Could you check a few things on this model? Use its own coordinates, in mm. A direction names the side the tool comes from. Coordinates: 2 decimals unless noted, no trailing zeros. Order: outer loops, then holes, each group sorted by start corner. A loop starts at its lowest first (then second) coordinate and runs counter-clockwise, first axis right, second up. Notation, with made-up numbers: M 62,39 L 87,39 A26 cw 87,74 Z; hole C 85.25,-4 d4. An arc over 180 degrees is marked long. One line per question, with ' | ' between items. Start each with the question number.
from build123d import *

# Parameters (mm, degrees)
CYLINDER157_R     = 2
CYLINDER157_DEPTH = 10
EXTRUDE038_DEPTH  = 28


with BuildPart() as cylinder157:
    # Cylinder157 → Cylinder157 (new body)
    with BuildSketch(Plane(origin=(0, -238, -147.25), x_dir=(1, 0, 0), z_dir=(0, -1, 0))):
        Circle(CYLINDER157_R)
    extrude(amount=CYLINDER157_DEPTH)


with BuildPart() as logoattach001:
    # Sketch056 → Extrude038 (new body)
    with BuildSketch(Plane.XY):
        with BuildLine():
            ThreePointArc((-20, -241.335918), (0, -243.5), (20, -241.335918))
            Line((20, -237.335918), (20, -241.335918))
            Line((-20, -237.335918), (20, -237.335918))
            Line((-20, -241.335918), (-20, -237.335918))
        make_face()
    extrude(amount=EXTRUDE038_DEPTH)


with BuildPart() as logoattach001_1:
    # Extrude038 placement: moved
    add(logoattach001.part.moved(Location((0, 0, -160))))

    # Fusion105: union Cylinder157
    add(cylinder157.part)


solid = logoattach001_1.part
(1) On a 3-axis mill with a long thin cutter (end or side, diameter ignored), from which of +Z, -Z, +X, -X, +Y, -Y can I reach the whole of each face in a straight line? I mean faces 1 (the flat face through (0, -240, -160)), 2 (the cylindrical face through (0.923, -245.707, -149.024)). Say none if no direction works.
(2) Imagine slicing it at B-B, the plane z = -147.25. Write out the boundary of the cut face in (x, y), plus the area to 3 significant figures.
(3) Imagine slicing it at A-A, the plane x = 0. Write out the boundary of the cut face in (y, z).
(4) For P1, Ø10, axis at x = -11, z = -139.5, coming from the -Y side; P2, Ø3, axis at y = -242.5, z = -146, coming from the +X side, each with a flat end and sliding along its axis, tell me the tip position at first contact or that it passes through.
(5) If I drill on line 1 along Y through (x, z) = (7.5, -138); line 2 along Y through (x, z) = (-9.5, -144.5); line 3 along Z through (x, y) = (0.5, -244), over which ranges is the centre line in solid material (lowest first)? Write a range as from..to.
(6) Imagine slicing it at C-C, the plane y = -244.5. Write out the boundary of the cut face in (x, z), plus the area to 3 significant figures.
(7) Imagine slicing it at D-D, the plane z = -155. Write out the boundary of the cut face in (x, y), plus the area to 3 significant figures.
Answers:
1) face 1: -Z, +X, -X, +Y, -Y | face 2: -Y
2) outline: M -20,-241.34 A93.5 ccw -2,-243.48 L -2,-248 L 2,-248 L 2,-243.48 A93.5 ccw 20,-241.34 L 20,-237.34 L -20,-237.34 Z | area: 236 mm²
3) outline: M -248,-149.25 L -243.5,-149.25 L -243.5,-160 L -237.34,-160 L -237.34,-132 L -243.5,-132 L -243.5,-145.25 L -248,-145.25 Z
4) P1: y = -243.31 | P2: x = 20
5) line 1: -243.2..-237.34 | line 2: -243.02..-237.34 | line 3: -149.19..-145.31
6) outline: C 0,-147.25 d4 | area: 12.6 mm²
7) outline: M -20,-241.34 A93.5 ccw 20,-241.34 L 20,-237.34 L -20,-237.34 Z | area: 218 mm²
